Autodesk Inventor part; units mm, degrees
ref_plane "1_2_XY" through (0, 0, 0) normal (1, 0, 0) x (0, 0, -1)
ref_plane "1_2_YZ" through (0, 0, 0) normal (0, 0, -1) x (0, 1, 0)
ref_plane "1_2_ZX" through (0, 0, 0) normal (0, 1, 0) x (1, 0, 0)
sketch "Sketch_1" plane through (0, 0, 0) normal (1, 0, 0) x (0, 1, 0)
  line L0 (0, -3) -> (0, 3)
  line L1 (8.5, 3) -> (3.5, 3)
  line L2 (3.5, 3) -> (3, 2.5)
  line L3 (3, 2.5) -> (3, -2.5)
  line L4 (3, -2.5) -> (3.5, -3)
  line L5 (3.5, -3) -> (8.5, -3)
  line L6 (8.5, -3) -> (9, -2.5)
  line L7 (9, -2.5) -> (9, 2.5)
  line L8 (9, 2.5) -> (8.5, 3)
revolve "Revolution1" add sketch "Sketch_1" angle 180 about axis through (0, 0, -3) along (0, 0, -1)
sketch "Sketch_2" plane through (0, 0, 0) normal (0, 0, 1) x (1, 0, 0)
  line L0 (-0.5, -9) -> (0.5, -9)
  line L1 (0.5, -9) -> (0.5, 9)
  line L2 (0.5, 9) -> (-0.5, 9)
  line L3 (-0.5, 9) -> (-0.5, -9)
extrude "Extrusion1" cut sketch "Sketch_2" along normal mid plane 6
sketch "Sketch_3" plane through (0, 0, 0) normal (0, 0, 1) x (1, 0, 0)
  line L0 (9, -6) -> (0, -6)
  line L1 (0, -6) -> (0, -4.55)
  line L2 (0, -4.55) -> (3, -4.55)
  line L3 (3, -4.55) -> (3, -3.55)
  line L4 (3, -3.55) -> (9, -3.55)
  line L5 (9, -3.55) -> (9, -6)
  line L6 (9, -6) -> (0, -6)
revolve "Revolution2" cut sketch "Sketch_3" angle 360 about axis through (9, -6, 0) along (-1, 0, 0)
sketch "Sketch_4" plane through (0, 0, 0) normal (0, 0, 1) x (1, 0, 0)
  line L0 (9, 6) -> (0, 6)
  line L1 (0, 6) -> (0, 7.45)
  line L2 (0, 7.45) -> (3, 7.45)
  line L3 (3, 7.45) -> (3, 8.45)
  line L4 (3, 8.45) -> (9, 8.45)
  line L5 (9, 8.45) -> (9, 6)
  line L6 (9, 6) -> (0, 6)
revolve "Revolution3" cut sketch "Sketch_4" angle 360 about axis through (9, 6, 0) along (-1, 0, 0)
ref_plane "1_2_XY" through (0, 0, 0) normal (1, 0, 0) x (0, 0, -1)
ref_plane "1_2_YZ" through (0, 0, 0) normal (0, 0, -1) x (0, 1, 0)
ref_plane "1_2_ZX" through (0, 0, 0) normal (0, 1, 0) x (1, 0, 0)
ref_plane "body_screw_XY" through (3, -6, 0) normal (1, 0, 0) x (0, 0, -1)
ref_plane "body_screw_YZ" through (3, -6, 0) normal (0, 0, -1) x (0, 1, 0)
ref_plane "body_screw_ZX" through (3, -6, 0) normal (0, 1, 0) x (1, 0, 0)
ref_plane "body_screw2_XY" through (3, 6, 0) normal (1, 0, 0) x (0, 0, -1)
ref_plane "body_screw2_YZ" through (3, 6, 0) normal (0, 0, -1) x (0, 1, 0)
ref_plane "body_screw2_ZX" through (3, 6, 0) normal (0, 1, 0) x (1, 0, 0)
properties part number "PSCSPJ6-6b"
Geometry check sheet. Reference: the model listing, model coordinates, mm. A direction names the side the tool comes from. Coordinates: 2 decimals unless noted, no trailing zeros. Loops run counter-clockwise (first coordinate to the right, second up) from the corner with the lowest first, then second, coordinate; pieces in that order, holes last.
Item 1: Release check for a two-part mould opening along Y. For faces 3 (the face through (5, 0, -3)), 4 (the face through (3, -6, 2)), 5 (the face through (8.64, 0.18, 2.86)) record: released by +Y, released by -Y, zero draft, split by the parting line, or undercut.
Item 2: Thickness scan on line 1 (Y direction, x = 2.2, z = 0); line 2 (Z direction, x = 4.75, y = -6); line 3 (X direction, y = -7.5, z = 1.5). Record the ranges inside material, lowest first.
Item 3: Sectioned sample at B-B, the plane z = 1. Record the boundary of the cut face in (x, y).
Item 4: Go/stop test with flat-tipped pins: pin 1 Ø2.5 at (y, z) = (5.5, 0.5) entering from +X; pin 2 Ø3 at (x, z) = (4.5, 2) entering from -Y; pin 3 Ø1.5 at (x, z) = (5.5, 2.5) entering from -Y. Record where each tip stops, or that it passes through.
Item 5: Sectioned sample at A-A, the plane y = 0. Record the boundary of the cut face in (x, z), then the cut area to 3 significant figures.
Item 6: Sectioned sample at D-D, the plane x = 2.75. Count the separate pieces of the cut face and the enclosed holes in it, then the cut area to 3 significant figures.
Item 7: Access from +Z, -Z, +X, -X, +Y, -Y to the whole of each face (thin tool, end or side, straight path). Record for faces 1 (the face through (3, 0, 0)), 2 (the face through (5.086, -3.663, 0.736)).
Item 8: Sectioned sample at C-C, the plane z = 2.25. Record the boundary of the cut face in (x, y).
Check result:
1. face 3: zero draft
1. face 4: undercut
1. face 5: split by the parting line
2. line 1: y = -8.73 to -7.45, -4.55 to -2.04, 2.04 to 4.55, 7.45 to 8.73
2. line 2: z = -3 to -2.45, 2.45 to 3
2. line 3: x = 0.5 to 3
3. outline: (0.5, -8.99) arc R9 ccw to (3.63, -8.24) - (3, -8.24) - (3, -7.05) - (0.5, -7.05) - close; (0.5, -4.95) - (3, -4.95) - (3, -3.76) - (8.18, -3.76) arc R9 ccw to (8.18, 3.76) - (3, 3.76) - (3, 4.95) - (0.5, 4.95) - (0.5, 2.96) arc R3 cw to (0.5, -2.96) - close; (0.5, 7.05) - (3, 7.05) - (3, 8.24) - (3.63, 8.24) arc R9 ccw to (0.5, 8.99) - close
4. pin 1: stops at x = 3
4. pin 2: stops at y = -8.49
4. pin 3: stops at y = -7.64
5. outline: (3, -2.5) - (3.5, -3) - (8.5, -3) - (9, -2.5) - (9, 2.5) - (8.5, 3) - (3.5, 3) - (3, 2.5) - close
5. area: 35.5 mm2
6. separate pieces: 2
6. enclosed holes: 2
6. area: 73.7 mm2
7. face 1: +Z, -Z, -X
7. face 2: +X
8. outline: (0.5, -8.99) arc R9 ccw to (5.69, -6.97) - (3, -6.97) - (3, -5.03) - (7.46, -5.03) arc R9 ccw to (7.46, 5.03) - (3, 5.03) - (3, 6.97) - (5.69, 6.97) arc R9 ccw to (0.5, 8.99) - (0.5, 2.96) arc R3 cw to (0.5, -2.96) - close
